from build123d import *

# Parameters (mm, degrees)
F0_R     = 2.667
F0_W     = 15.24
F0_H     = 32.258
F1_DEPTH = 4.7625
F2_DEPTH = 13.0175
F3_W     = 7.62
F3_H     = 32.258
F6_DEPTH = 32.258
F7_SIZE  = 1.905


with BuildPart() as f1:
    # F0 (on Top) → F1 (new body)
    with BuildSketch(Plane.XY):
        Polygon((-11.1125, -38.481), (0, -41.021), (11.1834268409, -38.481), (15.5575, 0), (11.1834268409, 38.481), (0, 41.021), (-11.1125, 38.481), (-15.5575, 0), align=None)
        with Locations((0, -32.385)):
            Circle(F0_R, mode=Mode.SUBTRACT)
        with Locations((-5.3975, 0)):
            Rectangle(F0_W, F0_H, mode=Mode.SUBTRACT)
        with Locations((0, 32.385)):
            Circle(F0_R, mode=Mode.SUBTRACT)
        with Locations((7.9375, 0)):
            Circle(F0_R, mode=Mode.SUBTRACT)
    extrude(amount=F1_DEPTH)

    # F0 (on Top) → F2 (join)
    with BuildSketch(Plane.XY):
        with Locations((-5.3975, 0)):
            Rectangle(F0_W, F0_H)
    extrude(amount=F2_DEPTH)

    # F3 (on face) → F4 (revolve)
    with BuildSketch(Plane.XY.offset(13.0175)):
        with Locations((-9.2075, 0)):
            Rectangle(F3_W, F3_H)
    revolve(axis=Axis((-5.3975, 0, 13.0175), (0, -1, 0)))

    # F5 (on face) → F6 (cut)
    with BuildSketch(Plane.XZ.offset(16.129)):
        with BuildLine():
            ThreePointArc((-2.2225, 13.0175), (-5.3975, 16.1925), (-8.5725, 13.0175))
            ThreePointArc((-8.5725, 13.0175), (-5.3975, 9.8425), (-2.2225, 13.0175))
        make_face()
    extrude(amount=-F6_DEPTH, mode=Mode.SUBTRACT)

    # F7
    f7_edges = [f1.edges().sort_by_distance(p)[0] for p in [
        (-2.667, -32.385, 4.7625),
        (5.2705, 0, 4.7625),
        (-2.667, 32.385, 4.7625),
    ]]
    chamfer(f7_edges, length=F7_SIZE)


solid = f1.part
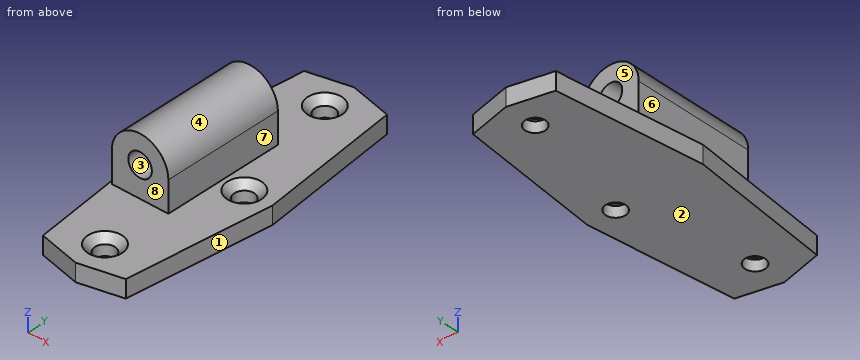
Design review of the part built by this model. Coordinates are the model's own, in mm. Face numbers are marked on the shaded views. A direction names the side the tool comes from. Give positions to 0.01 mm unless a question says otherwise; leave off trailing zeros. Write each loop counter-clockwise with the first axis right and the second up, starting at its lowest first coordinate (ties: lowest second). Pieces come first, ordered by that corner, then holes. Notation, with made-up numbers: M -14,-1.5 L 41,-1.5 A22 ccw 41,27.5 Z; hole C 16,25 d8. An arc over 180 degrees is marked long. Return JSON: item names as keys, results as strings. Group by question number.
Item 1: The part is to be moulded in two halves that separate along Z. For the marked faces 1, 2, 3 and 4, say which applies: pulls with the +Z half, pulls with the -Z half, needs draft (parallel to the pull), parting line crosses it, or undercut.
Item 2: Clearance check with flat-ended pins moving along their axes: pin 1 Ø3 at (x, y) = (7, -8.5) entering from +Z; pin 2 Ø12 at (x, z) = (-5, 12) entering from +Y; pin 3 Ø7 at (x, y) = (0, 32.385) entering from +Z. State where each tip first meets the part, or that it passes through.
Item 3: Take a section at B-B (z = 5.75). Give the boundary of the cut face in (x, y), plus the area to 3 significant figures.
Item 4: Tool access review of the marked faces 5, 6, 7 and 8: name each direction out of +Z, -Z, +X, -X, +Y, -Y from which nothing blocks a thin tool from reaching the whole face with its end or side.
Item 5: Take a section at C-C (y = 22). Give the boundary of the cut face in (x, z), plus the area to 3 significant figures.
Item 6: Wall thickness on line 1 along Y through (x, z) = (0, 2.2); line 2 along Z through (x, y) = (9.5, -12.5); line 3 along Y through (x, z) = (-9, 14): over which ranges is each line inside the solid? List them lowest first.
Return value:
{
 "1": {"face 1": "needs draft", "face 2": "pulls with the -Z half", "face 3": "undercut", "face 4": "pulls with the +Z half"},
 "2": {"pin 1": "stops at z = 4.76", "pin 2": "stops at y = 16.13", "pin 3": "stops at z = 3.69"},
 "3": {"outline": "M -13.02,-16.13 L 2.22,-16.13 L 2.22,16.13 L -13.02,16.13 Z", "area": "492 mm2"},
 "4": {"face 5": "+Z, +X, -X, +Y", "face 6": "+Z, -X, +Y, -Y", "face 7": "+Z, +X, +Y, -Y", "face 8": "+Z, +X, -X, -Y"},
 "5": {"outline": "M -13.02,0 L 13.06,0 L 13.06,4.76 L -13.02,4.76 Z", "area": "124 mm2"},
 "6": {"line 1": "y = -41.02 to -35.05, -29.72 to 29.72, 35.05 to 41.02", "line 2": "z = 0 to 4.76", "line 3": "y = -16.13 to 16.13"}
}
